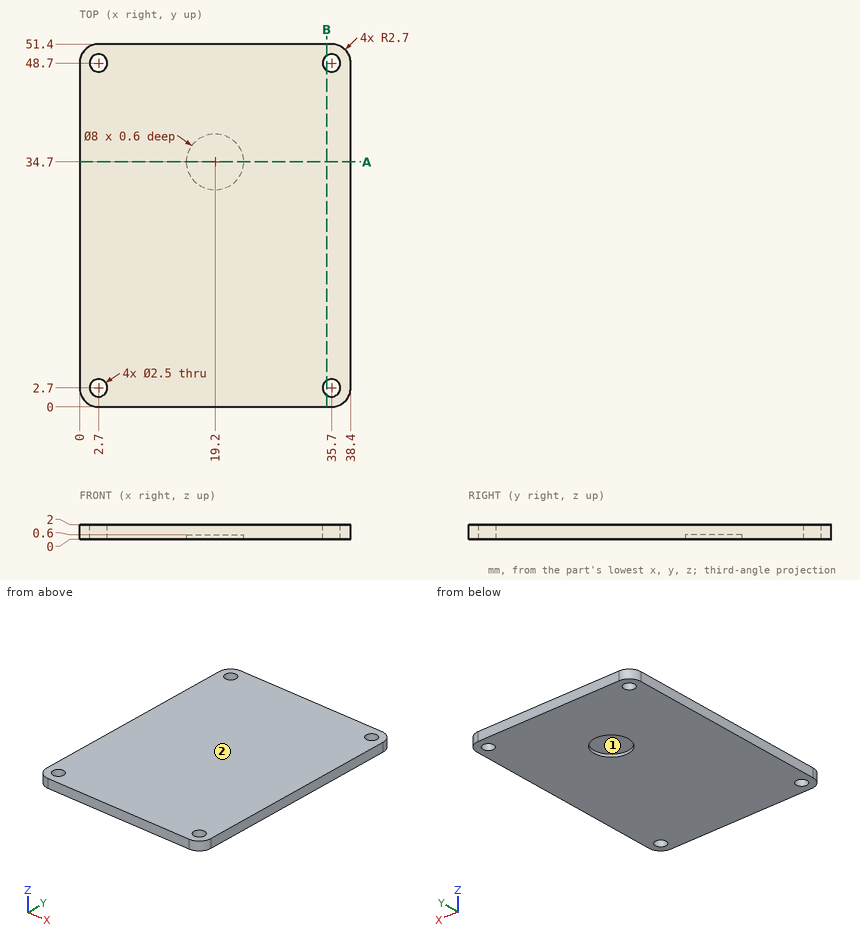
The drawing under review shows one solid part. Ordinate dimensions are in mm from its lowest x, y, z. Round coordinates to 2 decimals unless told otherwise and drop trailing zeros. Write each loop counter-clockwise with the first axis right and the second up, starting at its lowest first coordinate (ties: lowest second). Pieces come first, ordered by that corner, then holes. Notation, with made-up numbers: (-2, 7) - (54, 7) arc R10 ccw to (54, 15) - close; hole circle Ø3 at (42.25, 45.5). An arc over 180 degrees is marked (long way). Use a Markdown table: item, result. Add a question column.
1. Mouldability with a two-part tool opening along Y and no side actions: class the marked faces 1 and 2 as +Y half, -Y half, draft (parallel to the pull), parting line (faces both ways), or undercut.
2. Wall thickness on probe 1 along Y at (x, z) = (2.7, 1.5); probe 2 along X at (y, z) = (48, 0.85); probe 3 along X at (y, z) = (36, 0.2): over which ranges is each line inside the solid? List them lowest first.
3. Clearance check with a flat-ended pin moving along its axis: pin 1 (5 mm diameter, centred on x = 19.2, y = 34.7, fed in from -Z). State where the tip first meets the part, or that it passes through.
4. We need section B-B (x = 35). State the section outline as (y, z) points.
5. We need section A-A (y = 34.7). State the section outline as (x, z) points.
Output:
| question | item | result |
|---|---|---|
| 1 | face 1 | undercut |
| 1 | face 2 | draft |
| 2 | probe 1 | y = 0 to 1.45, 3.95 to 47.45, 49.95 to 51.4 |
| 2 | probe 2 | x = 0 to 1.66, 3.74 to 34.66, 36.74 to 38.4 |
| 2 | probe 3 | x = 0 to 15.42, 22.98 to 38.4 |
| 3 | pin 1 | stops at z = 0.6 |
| 4 | outline | (0, 0) - (1.66, 0) - (1.66, 2) - (0, 2) - close; (3.74, 0) - (47.66, 0) - (47.66, 2) - (3.74, 2) - close; (49.74, 0) - (51.4, 0) - (51.4, 2) - (49.74, 2) - close |
| 5 | outline | (0, 0) - (15.2, 0) - (15.2, 0.6) - (23.2, 0.6) - (23.2, 0) - (38.4, 0) - (38.4, 2) - (0, 2) - close |
